```python
from build123d import *

# Parameters (mm, degrees)
SKETCH1_W                       = 40.64
SKETCH1_H                       = 43.18
BOSS_EXTRUDE1_DEPTH             = 0.9144
SKETCH3_W                       = 5.08
SKETCH3_H                       = 5.08
BOSS_EXTRUDE2_DEPTH             = 1.27
SKETCH4_W                       = 12.7
SKETCH4_H                       = 25.654
BOSS_EXTRUDE3_DEPTH             = 4.064
F_32_0_116_DIAMETER_HOLE1_D     = 2.9464
F_32_0_116_DIAMETER_HOLE1_DEPTH = 25.4
F_32_0_116_DIAMETER_HOLE1_TIP   = 0.885187864


with BuildPart() as part:
    # Sketch1 → Boss-Extrude1 (new body)
    with BuildSketch(Plane(origin=(0, 0, 0), x_dir=(1, 0, 0), z_dir=(0, 1, 0))):
        with Locations((20.32, 21.59)):
            Rectangle(SKETCH1_W, SKETCH1_H)
    extrude(amount=BOSS_EXTRUDE1_DEPTH)

    # Sketch3 → Boss-Extrude2 (add)
    with BuildSketch(Plane(origin=(0, 0.9144, 0), x_dir=(1, 0, 0), z_dir=(0, 1, 0))):
        with Locations((20.32, 12.7)):
            Rectangle(SKETCH3_W, SKETCH3_H)
        with Locations((27.94, 12.7)):
            Rectangle(SKETCH3_W, SKETCH3_H)
        with Locations((27.94, 5.08)):
            Rectangle(SKETCH3_W, SKETCH3_H)
        with Locations((20.32, 5.08)):
            Rectangle(SKETCH3_W, SKETCH3_H)
    extrude(amount=BOSS_EXTRUDE2_DEPTH)

    # Sketch4 → Boss-Extrude3 (add)
    with BuildSketch(Plane(origin=(0, 0.9144, 0), x_dir=(1, 0, 0), z_dir=(0, 1, 0))):
        with Locations((6.985, 13.462)):
            Rectangle(SKETCH4_W, SKETCH4_H)
    extrude(amount=BOSS_EXTRUDE3_DEPTH)

    # #32 (0.116) Diameter Hole1
    with Locations(Plane(origin=(0, 0.9144, 0), x_dir=(1, 0, 0), z_dir=(0, 1, 0))):
        with Locations((3.81, 39.37), (36.83, 39.37), (36.83, 3.81), (15.24, 3.81)):
            Hole(F_32_0_116_DIAMETER_HOLE1_D / 2, depth=F_32_0_116_DIAMETER_HOLE1_DEPTH)
            with Locations((0, 0, -(F_32_0_116_DIAMETER_HOLE1_DEPTH + F_32_0_116_DIAMETER_HOLE1_TIP / 2))):  # 118° drill point
                Cone(0, F_32_0_116_DIAMETER_HOLE1_D / 2, F_32_0_116_DIAMETER_HOLE1_TIP, mode=Mode.SUBTRACT)


solid = part.part
```
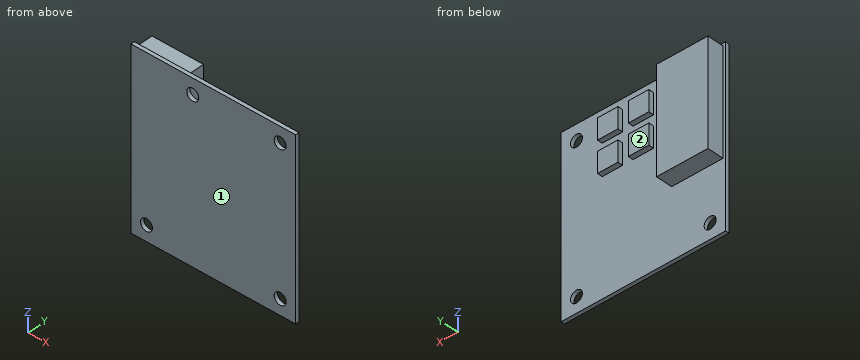
Geometry check sheet. Reference: the model listing, model coordinates, mm. Face numbers are marked on the shaded views. A direction names the side the tool comes from. Coordinates: 2 decimals unless noted, no trailing zeros. Loops run counter-clockwise (first coordinate to the right, second up) from the corner with the lowest first, then second, coordinate; pieces in that order, holes last. Notation, with made-up numbers: (57.5, -5) -> (105.5, -5) arc R21 cw to (105.5, 17) -> close; hole circle Ø5 at (27, 88). An arc over 180 degrees is marked (long way). Put each result on its own line as item: value.
1) Thickness scan on line 1 (X direction, y = 0.5, z = -4); line 2 (Z direction, x = 36.83, y = 0.45); line 3 (X direction, y = 0.5, z = -39.37). Record the ranges inside material, lowest first.
Result set:
line 1: x = 0 to 13.78, 16.7 to 35.37, 38.29 to 40.64
line 2: z = -43.18 to -40.84, -37.9 to -5.28, -2.34 to 0
line 3: x = 0 to 2.34, 5.28 to 35.36, 38.3 to 40.64
2) Cross-section at A-A on x = 3.81. Record the boundary of the cut face in (y, z) (3 decimals), plus the area to 3 significant figures.
Result set:
outline: (0, -43.18) -> (0.914, -43.18) -> (0.914, -40.843) -> (0, -40.843) -> close; (0, -37.897) -> (0.914, -37.897) -> (0.914, -26.289) -> (4.978, -26.289) -> (4.978, -0.635) -> (0.914, -0.635) -> (0.914, 0) -> (0, 0) -> close
area: 141 mm^2
3) Cross-section at B-B on z = -39.37. Record the boundary of the cut face in (x, y), plus the area to 3 significant figures.
Result set:
outline: (0, 0) -> (2.34, 0) -> (2.34, 0.91) -> (0, 0.91) -> close; (5.28, 0) -> (35.36, 0) -> (35.36, 0.91) -> (5.28, 0.91) -> close; (38.3, 0) -> (40.64, 0) -> (40.64, 0.91) -> (38.3, 0.91) -> close
area: 31.8 mm^2
4) Gauge pin test, flat ends, axial feed: pin 1 Ø4 at (x, z) = (20.5, -13.5) entering from +Y; pin 2 Ø0.6 at (x, y) = (21.5, 1.5) entering from -Z; pin 3 Ø2 at (x, z) = (29, -16.5) entering from +Y. Record the tip position at first contact, or that the pin passes through.
Result set:
pin 1: stops at y = 2.18
pin 2: stops at z = -15.24
pin 3: stops at y = 0.91
5) Cross-section at C-C on x = 36.83. Record the boundary of the cut face in (y, z).
Result set:
outline: (0, -43.18) -> (0.91, -43.18) -> (0.91, -40.84) -> (0, -40.84) -> close; (0, -37.9) -> (0.91, -37.9) -> (0.91, -5.28) -> (0, -5.28) -> close; (0, -2.34) -> (0.91, -2.34) -> (0.91, 0) -> (0, 0) -> close
6) Tool access check on the marked faces 1 and 2. Record the directions out of +Z, -Z, +X, -X, +Y, -Y that give a thin tool (end or side, any length) a straight path to the whole face; none if there is none.
Result set:
face 1: +Z, -Z, +X, -X, -Y
face 2: +Z, -Z, +X, +Y
7) Cross-section at D-D on z = -13. Record the boundary of the cut face in (x, y) (3 decimals).
Result set:
outline: (0, 0) -> (40.64, 0) -> (40.64, 0.914) -> (30.48, 0.914) -> (30.48, 2.184) -> (25.4, 2.184) -> (25.4, 0.914) -> (22.86, 0.914) -> (22.86, 2.184) -> (17.78, 2.184) -> (17.78, 0.914) -> (13.335, 0.914) -> (13.335, 4.978) -> (0.635, 4.978) -> (0.635, 0.914) -> (0, 0.914) -> close
